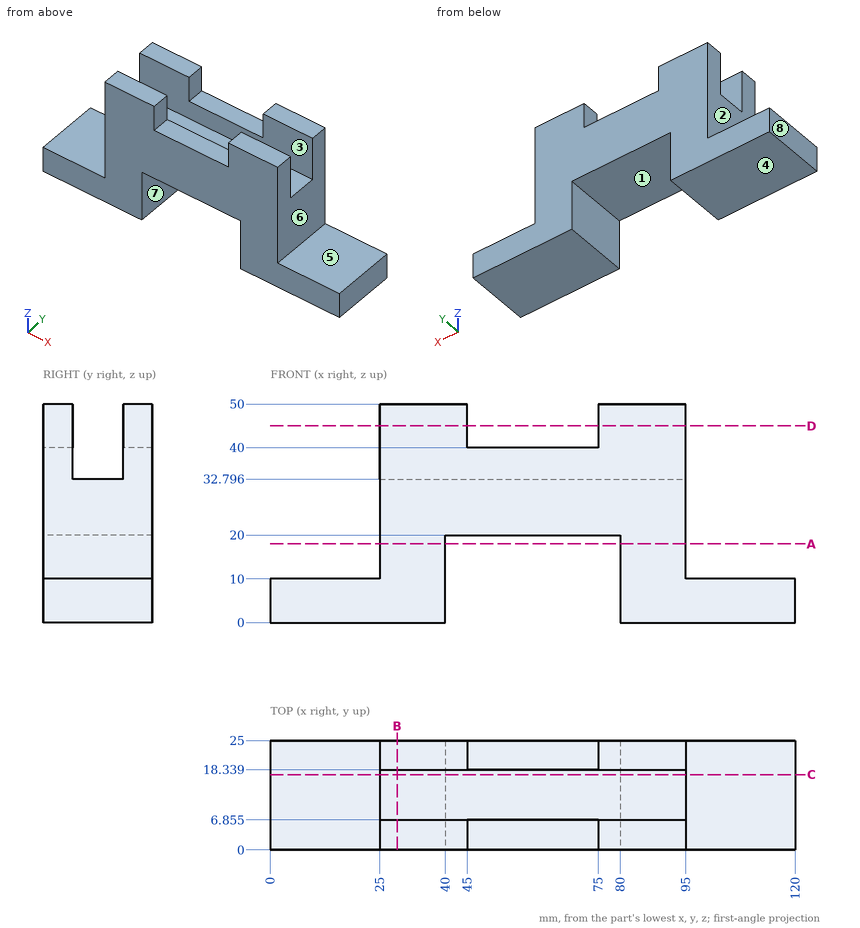
Can you work these out from the drawing? Everything is in mm from the part's minimum corner. A direction names the side the tool comes from. Round coordinates to 2 decimals unless told otherwise and drop trailing zeros. Loops run counter-clockwise (first coordinate to the right, second up) from the corner with the lowest first, then second, coordinate; pieces in that order, holes last. Notation, with made-up numbers: (25.25, 67) -> (36.25, 67) arc R16 ccw to (36.25, 89) -> close; hole circle Ø4 at (42, -10). An arc over 180 degrees is marked (long way). One line per question, with ' | ' between items.
(1) If we section it at C-C on y = 17.25: List the corners of the cut face in (x, z) for me, and give its area (3 significant figures).
Model answer:
outline: (0, 0) -> (40, 0) -> (40, 20) -> (80, 20) -> (80, 0) -> (120, 0) -> (120, 10) -> (95, 10) -> (95, 32.8) -> (25, 32.8) -> (25, 10) -> (0, 10) -> close | area: 2,000 mm^2
(2) If we section it at B-B on x = 29: List the corners of the cut face in (y, z) for me (1 decimal).
Model answer:
outline: (0, 0) -> (25, 0) -> (25, 50) -> (18.3, 50) -> (18.3, 32.8) -> (6.9, 32.8) -> (6.9, 50) -> (0, 50) -> close
(3) For pin 1 Ø2 at (y, z) = (22, 44.5) entering from +X; pin 2 Ø3.5 at (y, z) = (2.5, 46) entering from -X; pin 3 Ø7.5 at (x, y) = (106, 16.5) entering from +Z, each with a flat end and sliding along its axis, tell me the tip position at first contact or that it passes through.
Model answer:
pin 1: stops at x = 95 | pin 2: stops at x = 25 | pin 3: stops at z = 10
(4) If I drill on probe 1 along X at (y, z) = (3.75, 11); probe 2 along X at (y, z) = (4.5, 42); probe 3 along Y at (x, z) = (91.5, 33.5) (1 decimal), over which ranges is the centre line in solid material (lowest first)?
Model answer:
probe 1: x = 25 to 40, 80 to 95 | probe 2: x = 25 to 45, 75 to 95 | probe 3: y = 0 to 6.9, 18.3 to 25
(5) For the marked faces 1, 2, 3, 4 and 5, which set-ups out of +Z, -Z, +X, -X, +Y, -Y let a thin tool reach every point of the face, with its end or its side?
Model answer:
face 1: -Z, +Y, -Y | face 2: +Z, -X, +Y, -Y | face 3: +Z, +X, -X | face 4: -Z, +X, -X, +Y, -Y | face 5: +Z, +X, +Y, -Y
(6) If we section it at A-A on z = 18: List the corners of the cut face in (x, y) for me, and give its area (3 significant figures).
Model answer:
outline: (25, 0) -> (40, 0) -> (40, 25) -> (25, 25) -> close; (80, 0) -> (95, 0) -> (95, 25) -> (80, 25) -> close | area: 750 mm^2
(7) Thinking about a two-plate mould opening in X: for the marked faces 6, 7 and 8, which applies, released by +X, released by -X, zero draft, split by the parting line, or undercut?
Model answer:
face 6: released by +X | face 7: undercut | face 8: released by -X
(8) If we section it at D-D on z = 45: List the corners of the cut face in (x, y) for me (1 decimal).
Model answer:
outline: (25, 0) -> (45, 0) -> (45, 6.9) -> (25, 6.9) -> close; (25, 18.3) -> (45, 18.3) -> (45, 25) -> (25, 25) -> close; (75, 0) -> (95, 0) -> (95, 6.9) -> (75, 6.9) -> close; (75, 18.3) -> (95, 18.3) -> (95, 25) -> (75, 25) -> close
